Can you work these out from the model? Positions are in its coordinate system, mm. Face numbers are marked on the shaded views. A direction names the side the tool comes from. Give positions to 0.01 mm unless a question says otherwise; leave off trailing zeros. Loops run counter-clockwise (first coordinate to the right, second up) from the corner with the lowest first, then second, coordinate; pieces in that order, holes last.
from build123d import *

# Parameters (mm, degrees)
SKETCH_1_W           = 10
SKETCH_1_H           = 6
EXTRUDE_1_DEPTH      = 7
SKETCH_2_W           = 8.6
SKETCH_2_H           = 4.6
CUT_EXTRUDE_1_DEPTH  = 5
CUT_EXTRUDE_2_REACH  = 15.601
SKETCH_3_W           = 1
SKETCH_3_H           = 4
SKETCH_4_W           = 4
SKETCH_4_H           = 1
CUT_EXTRUDE_3_DEPTH  = 14.601470509
EXTRUDE_2_DEPTH      = 4
EXTRUDE_2_DEPTH_BACK = 4
SKETCH_5_R           = 0.4
FILLET_1_R           = 0.4


with BuildPart() as part:
    # 草图1 → 凸台-拉伸1 (new body)
    with BuildSketch(Plane.XY):
        with Locations((5, 3)):
            Rectangle(SKETCH_1_W, SKETCH_1_H)
    extrude(amount=EXTRUDE_1_DEPTH)

    # 草图2 → 切除-拉伸1 (cut)
    with BuildSketch(Plane.XY):
        with Locations((5, 3)):
            Rectangle(SKETCH_2_W, SKETCH_2_H)
    extrude(amount=CUT_EXTRUDE_1_DEPTH, mode=Mode.SUBTRACT)

    # 草图3 → 切除-拉伸2 (cut, up to next)
    with BuildSketch(Plane(origin=(0, 6, 0), x_dir=(1, 0, 0), z_dir=(0, 1, 0)), mode=Mode.PRIVATE) as cut_extrude_2_sk1:
        with Locations((6.99408033, -2)):
            Rectangle(SKETCH_3_W, SKETCH_3_H)
    cut_extrude_2_tool1 = extrude(cut_extrude_2_sk1.sketch, amount=-CUT_EXTRUDE_2_REACH, mode=Mode.PRIVATE) & part.part
    # 草图3 → 切除-拉伸2 (cut, up to next)
    with BuildSketch(Plane(origin=(0, 6, 0), x_dir=(1, 0, 0), z_dir=(0, 1, 0)), mode=Mode.PRIVATE) as cut_extrude_2_sk2:
        with Locations((2.99408033, -2)):
            Rectangle(SKETCH_3_W, SKETCH_3_H)
    cut_extrude_2_tool2 = extrude(cut_extrude_2_sk2.sketch, amount=-CUT_EXTRUDE_2_REACH, mode=Mode.PRIVATE) & part.part
    add(cut_extrude_2_tool1.solids().sort_by_distance((6.99408, 6, 2))[0], mode=Mode.SUBTRACT)
    add(cut_extrude_2_tool2.solids().sort_by_distance((2.99408, 6, 2))[0], mode=Mode.SUBTRACT)

    # 草图4 → 切除-拉伸3 (cut, through all)
    with BuildSketch(Plane(origin=(10, 0, 0), x_dir=(0, 0, -1), z_dir=(1, 0, 0))):
        with Locations((-2, 4.8)):
            Rectangle(SKETCH_4_W, SKETCH_4_H)
    extrude(amount=-CUT_EXTRUDE_3_DEPTH, mode=Mode.SUBTRACT)

    # 草图5 → 凸台-拉伸2 (add, two sides: drawn at the far end of the back side and taken through both)
    with BuildSketch(Plane(origin=(0, 0, 5), x_dir=(-1, 0, 0), z_dir=(0, 0, -1)).offset(-EXTRUDE_2_DEPTH_BACK)):
        with Locations((-5, 4)):
            Circle(SKETCH_5_R)
        with Locations((-7.5, 4)):
            Circle(SKETCH_5_R)
        with Locations((-2.5, 4)):
            Circle(SKETCH_5_R)
    extrude(amount=EXTRUDE_2_DEPTH + EXTRUDE_2_DEPTH_BACK)

    # 圆角1
    fillet_1_edges = [part.edges().sort_by_distance(p)[0] for p in [
        (2.9, 4, 9),
        (2.9, 4, 1),
        (5.4, 4, 9),
        (5.4, 4, 1),
        (7.9, 4, 9),
        (7.9, 4, 1),
    ]]
    fillet(fillet_1_edges, radius=FILLET_1_R)


solid = part.part
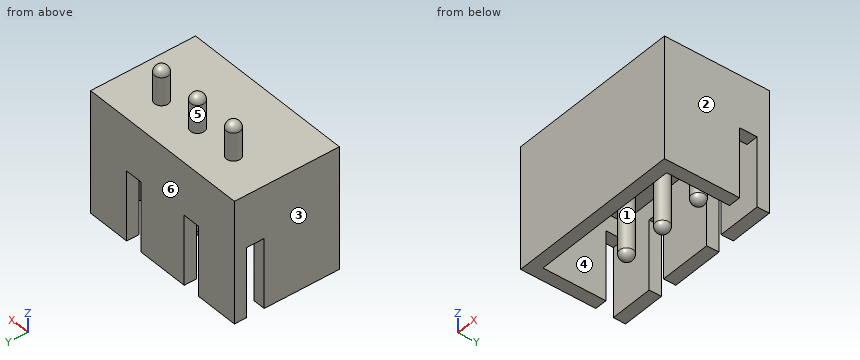
(1) Suppose I cut it at D-D on x = 5. List the corners of the cut face in (y, z) for me, plus the area to 3 significant figures.
Returned:
outline: (0, 0) - (0.7, 0) - (0.7, 5) - (3.6, 5) - (3.6, 1.4) arc R0.4 ccw to (4.4, 1.4) - (4.4, 5) - (5.3, 5) - (5.3, 0) - (6, 0) - (6, 7) - (4.4, 7) - (4.4, 8.6) arc R0.4 ccw to (3.6, 8.6) - (3.6, 7) - (0, 7) - close
area: 23.7 mm2
(2) Please list where these lines run through material, in increasing order: probe 1 along X at (y, z) = (5.4, 3); probe 2 along Y at (x, z) = (6, 4.75); probe 3 along X at (y, z) = (4.45, 4.5).
Returned:
probe 1: x = 0 to 2.49, 3.49 to 6.49, 7.49 to 10
probe 2: y = 0 to 0.7, 5.3 to 6
probe 3: x = 0 to 0.7, 9.3 to 10
(3) Suppose I cut it at A-A on z = 4.25. List the corners of the cut face in (x, y) for me, plus the area to 3 significant figures.
Returned:
outline: (0, 0) - (10, 0) - (10, 6) - (0, 6) - close; circle Ø0.8 at (2.5, 4); circle Ø0.8 at (5, 4); circle Ø0.8 at (7.5, 4); hole (0.7, 0.7) - (9.3, 0.7) - (9.3, 5.3) - (0.7, 5.3) - close
area: 21.9 mm2
(4) Suppose I cut it at B-B on z = 1.75. List the corners of the cut face in (x, y) for me.
Returned:
outline: (0, 0) - (10, 0) - (10, 4.3) - (9.3, 4.3) - (9.3, 0.7) - (0.7, 0.7) - (0.7, 4.3) - (0, 4.3) - close; (0, 5.3) - (2.49, 5.3) - (2.49, 6) - (0, 6) - close; circle Ø0.8 at (2.5, 4); (3.49, 5.3) - (6.49, 5.3) - (6.49, 6) - (3.49, 6) - close; circle Ø0.8 at (5, 4); circle Ø0.8 at (7.5, 4); (7.49, 5.3) - (10, 5.3) - (10, 6) - (7.49, 6) - close
(5) Which directions (+Z, -Z, +X, -X, +Y, -Y) give clear straight access to the entire face, cutting with the end or side of a thin tool? Please do the marked faces 4, 5 and 6.
Returned:
face 4: -Z
face 5: +Z
face 6: +Z, -Z, +X, -X, +Y
(6) Thinking about a two-plate mould opening in X: for the marked faces 1, 2 and 3, which applies, pulls with the +X half, pulls with the -X half, needs draft (parallel to the pull), parting line crosses it, or undercut?
Returned:
face 1: undercut
face 2: pulls with the +X half
face 3: pulls with the -X half
